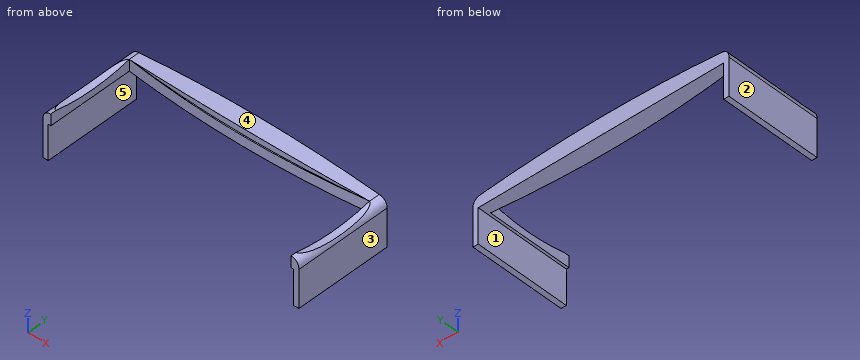
```python
from build123d import *

# Parameters (mm, degrees)
BOSS_EXTRUDE1_DEPTH     = 55
CUT_EXTRUDE1_DEPTH      = 95.637466314
CUT_EXTRUDE1_DEPTH_BACK = 95.637466314
CUT_EXTRUDE2_DEPTH      = 158.489682338
CUT_EXTRUDE2_DEPTH_BACK = 158.489682338
SKETCH4_W               = 3
SKETCH4_H               = 55
BOSS_EXTRUDE2_DEPTH     = 10


with BuildPart() as part:
    # Sketch1 → Boss-Extrude1 (new body)
    with BuildSketch(Plane(origin=(0, 0, 0), x_dir=(1, 0, 0), z_dir=(0, 1, 0))):
        with BuildLine():
            Line((-73.5, 3), (-73.5, 13))
            Line((-73.5, 13), (-70.5, 13))
            Line((-70.5, 13), (-70.5, 3))
            Line((-70.5, 3), (70.5, 3))
            Line((70.5, 3), (70.5, 13))
            Line((70.5, 13), (73.5, 13))
            Line((73.5, 13), (73.5, 3))
            Line((73.5, 3), (73.5, -3))
            ThreePointArc((73.5, -3), (0, -7), (-73.5, -3))
            Line((-73.5, -3), (-73.5, 3))
        make_face()
    extrude(amount=BOSS_EXTRUDE1_DEPTH)

    # Fillet1
    # a fillet whose section is not a circle: 5 mm, written as the material it takes off along each edge
    with BuildSketch(Plane(origin=(73.5, -11.289002285, 3), x_dir=(0, 0, -1), z_dir=(0, 1, 0))) as fillet1_piece_1:
        with BuildLine():
            Bezier((4.498901921, 0), (-0.015132067, 0), (-0.475075473, 4.490540603), weights=[1, 1, 1])
            ThreePointArc((-0.475075473, 4.490540603), (-0.24128019, 2.24487437), (0, 0))
            Line((0, 0), (4.498901921, 0))
        make_face()
    extrude(amount=77.578004571, mode=Mode.SUBTRACT)
    with BuildSketch(Plane(origin=(-73.5, -11.289002285, 3), x_dir=(0, 0, -1), z_dir=(0, 1, 0))) as fillet1_piece_2:
        with BuildLine():
            Bezier((4.498901921, 0), (-0.015132067, 0), (-0.475075473, -4.490540603), weights=[1, 1, 1])
            ThreePointArc((-0.475075473, -4.490540603), (-0.24128019, -2.24487437), (0, 0))
            Line((0, 0), (4.498901921, 0))
        make_face()
    extrude(amount=77.578004571, mode=Mode.SUBTRACT)

    # Sketch2 → Cut-Extrude1 (cut, two sides: drawn at the far end of the back side and taken through both)
    with BuildSketch(Plane.XY.offset(10).offset(-CUT_EXTRUDE1_DEPTH_BACK)):
        with BuildLine():
            Line((-69.009459397, 49), (-69.009459397, 0))
            Line((-69.009459397, 0), (69.009459397, 0))
            Line((69.009459397, 0), (69.009459397, 49))
            ThreePointArc((69.009459397, 49), (0, 45), (-69.009459397, 49))
        make_face()
    extrude(amount=CUT_EXTRUDE1_DEPTH + CUT_EXTRUDE1_DEPTH_BACK, mode=Mode.SUBTRACT)

    # Sketch3 → Cut-Extrude2 (cut, two sides: drawn at the far end of the back side and taken through both)
    with BuildSketch(Plane.ZY.offset(73.5).offset(-CUT_EXTRUDE2_DEPTH_BACK)):
        with BuildLine():
            Line((3.475075473, 49), (3.475075473, 3))
            ThreePointArc((3.475075473, 3), (0.975075473, 26), (3.475075473, 49))
        make_face()
    extrude(amount=CUT_EXTRUDE2_DEPTH + CUT_EXTRUDE2_DEPTH_BACK, mode=Mode.SUBTRACT)

    # Sketch4 → Boss-Extrude2 (add)
    with BuildSketch(Plane(origin=(0, 0, -13), x_dir=(-1, 0, 0), z_dir=(0, 0, -1))):
        with Locations((72, 27.5)):
            Rectangle(SKETCH4_W, SKETCH4_H)
        with Locations((-72, 27.5)):
            Rectangle(SKETCH4_W, SKETCH4_H)
    extrude(amount=BOSS_EXTRUDE2_DEPTH)


solid = part.part
```
Source: CAD feature listing. Evaluate the final solid. Frame: model axes, mm. Face numbers are marked on the shaded views. A direction names the side the tool comes from. Give positions to 0.01 mm unless a question says otherwise; leave off trailing zeros. Loops run counter-clockwise (first coordinate to the right, second up) from the corner with the lowest first, then second, coordinate; pieces in that order, holes last. Notation, with made-up numbers: (75, 22) -> (131, 22) arc R20 ccw to (131, 45) -> close; hole circle Ø3 at (27, 29.25). An arc over 180 degrees is marked (long way). Use a Markdown table: item, result. Add a question column.
(1) First-contact query: pin 1 Ø7 at (y, z) = (36.5, 1.5) entering from +X; pin 2 Ø1.2 at (x, y) = (7, 47.5) entering from -Z. Flat tips, straight axial feed; report the tip coordinate or a pass-through.
(2) Section query A-A (z = -6). Output: boundary loops of the cut face in (x, y), then the cut area to 3 significant figures.
(3) Access query for the marked faces 4 and 5. Directions: +Z, -Z, +X, -X, +Y, -Y. A direction counts if a zero-diameter tool reaches every point of the face in a straight line with its end or side. Return the directions, or none.
(4) Section query B-B (x = 54.5). Output: boundary loops of the cut face in (y, z), then the cut area to 3 significant figures.
(5) Pull-direction query (X, two-part tool) for the marked faces 1, 2 and 3; classes: +X half, -X half, draft (parallel to the pull), parting line (faces both ways), or undercut.
(6) Section query C-C (x = 28). Output: boundary loops of the cut face in (y, z), then the cut area to 3 significant figures.
(7) Ray query, line 1 (X direction, y = 4, z = -8.5); line 2 (Z direction, x = 3.5, y = 51); line 3 (Y direction, x = 36, z = -0.5). Return the intervals inside material, ascending.
Checked values:
| question | item | result |
|---|---|---|
| 1 | pin 1 | x = 73.5 |
| 1 | pin 2 | z = -3 |
| 2 | outline | (-73.5, 0) -> (-70.5, 0) -> (-70.5, 55) -> (-73.5, 55) -> close; (70.5, 0) -> (73.5, 0) -> (73.5, 55) -> (70.5, 55) -> close |
| 2 | area | 330 mm^2 |
| 3 | face 4 | +Z, +Y, -Y |
| 3 | face 5 | -Z, +Y, -Y |
| 4 | outline | (47.49, -3) -> (55, -3) -> (55, 4.8) -> (47.49, 4.8) -> (47.49, 3.48) -> (49, 3.48) arc R107.05 cw to (47.49, 3.15) -> close |
| 4 | area | 58.3 mm^2 |
| 5 | face 1 | undercut |
| 5 | face 2 | -X half |
| 5 | face 3 | +X half |
| 6 | outline | (45.66, -3) -> (55, -3) -> (55, 6.42) -> (45.66, 6.42) -> (45.66, 3.48) -> (49, 3.48) arc R107.05 cw to (45.66, 2.8) -> close |
| 6 | area | 86.9 mm^2 |
| 7 | line 1 | -73.5 to -70.5, 70.5 to 73.5 |
| 7 | line 2 | -3 to 6.99 |
| 7 | line 3 | 46.09 to 55 |
